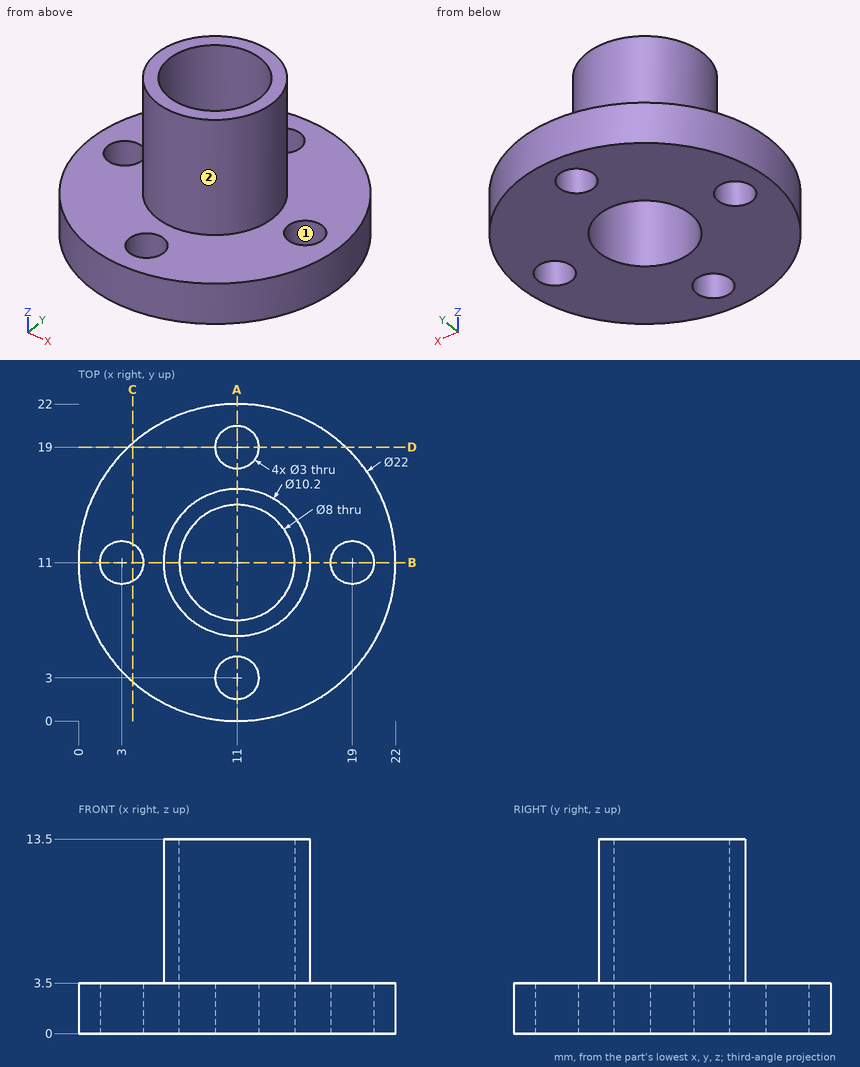
Geometry: see drawing. Coordinates: mm, zero at the bounding-box minimum. A direction names the side the tool comes from. Coordinates: 2 decimals unless noted, no trailing zeros. Order: outer loops, then holes, each group sorted by start corner. A loop starts at its lowest first (then second) coordinate and runs counter-clockwise, first axis right, second up. Notation, with made-up numbers: (61, 76.25) - (77, 76.25) arc R14 ccw to (77, 92.25) - close; hole circle Ø7 at (30.5, 31). An arc over 180 degrees is marked (long way). Write each question's results on one line, items separated by ' | '.
(1) Section query D-D, the plane y = 19. Return the cut outline in (x, z), plus the area to 3 significant figures.
Values found:
outline: (3.45, 0) - (9.5, 0) - (9.5, 3.5) - (3.45, 3.5) - close; (12.5, 0) - (18.55, 0) - (18.55, 3.5) - (12.5, 3.5) - close | area: 42.3 mm²
(2) Section query A-A, the plane x = 11. Return the cut outline in (y, z).
Values found:
outline: (0, 0) - (1.5, 0) - (1.5, 3.5) - (0, 3.5) - close; (4.5, 0) - (7, 0) - (7, 13.5) - (5.9, 13.5) - (5.9, 3.5) - (4.5, 3.5) - close; (15, 0) - (17.5, 0) - (17.5, 3.5) - (16.1, 3.5) - (16.1, 13.5) - (15, 13.5) - close; (20.5, 0) - (22, 0) - (22, 3.5) - (20.5, 3.5) - close
(3) Line query: line 1 (Y direction, x = 11, z = 4.75); line 2 (Z direction, x = 20.75, y = 14); line 3 (Y direction, x = 14, z = 12.75). Output: solid intervals per line, ascending. Write a range as [from, to].
Values found:
line 1: y = [5.9, 7], [15, 16.1] | line 2: z = [0, 3.5] | line 3: y = [6.88, 8.35], [13.65, 15.12]
(4) First-contact query: pin 1 Ø1.8 at (x, y) = (11, 3) entering from +Z; pin 2 Ø1 at (y, z) = (14, 5.5) entering from -X; pin 3 Ø1.5 at (x, z) = (14.5, 4.5) entering from +Y; pin 4 Ø3 at (x, z) = (12, 10.5) entering from +Y. Flat tips, straight axial feed; report the tip coordinate or a pass-through.
Values found:
pin 1: passes through | pin 2: stops at x = 6.55 | pin 3: stops at y = 15.3 | pin 4: stops at y = 16.1
(5) Set-up query: the marked faces 1 and 2. Return all of +Z, -Z, +X, -X, +Y, -Y with unobstructed straight access to the full face (end or side cutting, diameter ignored); none if empty.
Values found:
face 1: +Z, -Z | face 2: +Z
(6) Section query C-C, the plane x = 3.75. Return the cut outline in (y, z).
Values found:
outline: (2.73, 0) - (9.7, 0) - (9.7, 3.5) - (2.73, 3.5) - close; (12.3, 0) - (19.27, 0) - (19.27, 3.5) - (12.3, 3.5) - close
